Job drawing, mm, ordinate dimensions from the low corner. One solid piece. Coordinates: 2 decimals unless noted, no trailing zeros. Order: outer loops, then holes, each group sorted by start corner. A loop starts at its lowest first (then second) coordinate and runs counter-clockwise, first axis right, second up. Notation, with made-up numbers: (17, -2) - (40, -2) arc R11 cw to (40, 19) - close; hole circle Ø4 at (89, 76). An arc over 180 degrees is marked (long way). Use a Markdown table: item, result. Add a question column.
1) Drop a flat-ended pin along its axis: P1, Ø4.5, axis at x = 4.5, y = 35, coming from the -Z side. Give the stop position or say it passes through.
2) Saw through at D-D on y = 14.5. List the corners of the cut face in (x, z), then the cut area to 3 significant figures.
3) Wall check: L1, parallel to Y at x = 4.5, z = 1.4; L2, parallel to X at y = 6, z = 0.95; L3, parallel to X at y = 44.5, z = 0.8. Give the ranges that are in metal, low to high. Write a range as [from, to].
4) Saw through at C-C on z = 0.75. List the corners of the cut face in (x, y).
5) Saw through at B-B on x = 4.5. List the corners of the cut face in (y, z), then the cut area to 3 significant figures.
6) Saw through at A-A on y = 35. List the corners of the cut face in (x, z).
7) Two-plate mould, pull along Y, no slides. Class the marked faces 1, 2, 3 and 4: +Y half, -Y half, draft (parallel to the pull), parting line (faces both ways), or undercut.
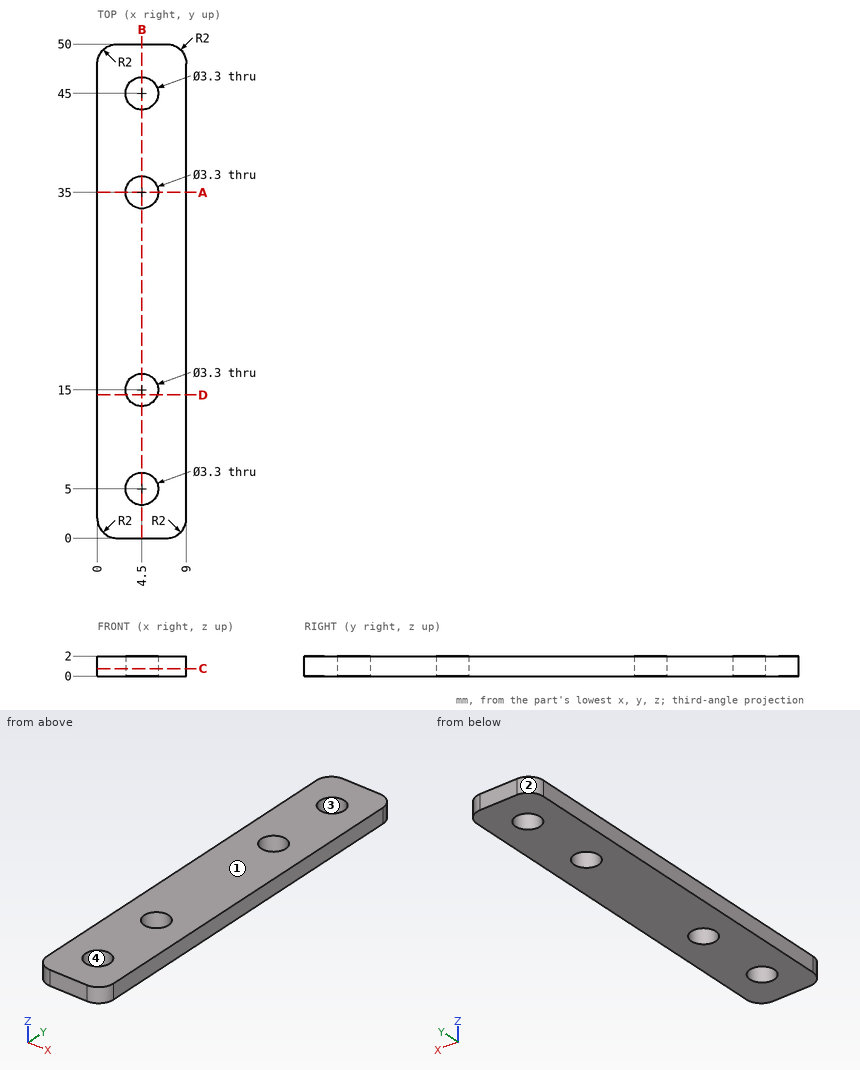
Results are:
| question | item | result |
|---|---|---|
| 1 | P1 | z = 0 |
| 2 | outline | (0, 0) - (2.93, 0) - (2.93, 2) - (0, 2) - close; (6.07, 0) - (9, 0) - (9, 2) - (6.07, 2) - close |
| 2 | area | 11.7 mm2 |
| 3 | L1 | [0, 3.35], [6.65, 13.35], [16.65, 33.35], [36.65, 43.35], [46.65, 50] |
| 3 | L2 | [0, 3.19], [5.81, 9] |
| 3 | L3 | [0, 2.93], [6.07, 9] |
| 4 | outline | (0, 2) arc R2 ccw to (2, 0) - (7, 0) arc R2 ccw to (9, 2) - (9, 48) arc R2 ccw to (7, 50) - (2, 50) arc R2 ccw to (0, 48) - close; hole circle Ø3.3 at (4.5, 5); hole circle Ø3.3 at (4.5, 15); hole circle Ø3.3 at (4.5, 35); hole circle Ø3.3 at (4.5, 45) |
| 5 | outline | (0, 0) - (3.35, 0) - (3.35, 2) - (0, 2) - close; (6.65, 0) - (13.35, 0) - (13.35, 2) - (6.65, 2) - close; (16.65, 0) - (33.35, 0) - (33.35, 2) - (16.65, 2) - close; (36.65, 0) - (43.35, 0) - (43.35, 2) - (36.65, 2) - close; (46.65, 0) - (50, 0) - (50, 2) - (46.65, 2) - close |
| 5 | area | 73.6 mm2 |
| 6 | outline | (0, 0) - (2.85, 0) - (2.85, 2) - (0, 2) - close; (6.15, 0) - (9, 0) - (9, 2) - (6.15, 2) - close |
| 7 | face 1 | draft |
| 7 | face 2 | +Y half |
| 7 | face 3 | undercut |
| 7 | face 4 | undercut |
